from build123d import *

# Parameters (mm, degrees)
SKETCH1_W           = 508
SKETCH1_H           = 546.1
BOSS_EXTRUDE1_DEPTH = 1.6002
SKETCH2_R           = 6.35
CUT_EXTRUDE1_DEPTH  = 2.54
SKETCH3_R           = 3.2639
CUT_EXTRUDE3_DEPTH  = 373.927423422
SKETCH4_R           = 6.35
CUT_EXTRUDE4_DEPTH  = 2.54


with BuildPart() as part:
    # Sketch1 → Boss-Extrude1 (new body)
    with BuildSketch(Plane(origin=(0, 0, 0), x_dir=(1, 0, 0), z_dir=(0, 1, 0))):
        Rectangle(SKETCH1_W, SKETCH1_H)
    extrude(amount=BOSS_EXTRUDE1_DEPTH)

    # Sketch2 → Cut-Extrude1 (cut)
    with BuildSketch(Plane(origin=(0, 1.6002, 0), x_dir=(1, 0, 0), z_dir=(0, 1, 0))):
        with Locations(Location((215.9, 222.25, 0), (0, 0, 270))):
            Circle(SKETCH2_R)
        with Locations(Location((215.9, -171.45, 0), (0, 0, 270))):
            Circle(SKETCH2_R)
        with Locations(Location((-215.9, 222.25, 0), (0, 0, 270))):
            Circle(SKETCH2_R)
        with Locations(Location((-215.9, -171.45, 0), (0, 0, 270))):
            Circle(SKETCH2_R)
    extrude(amount=-CUT_EXTRUDE1_DEPTH, mode=Mode.SUBTRACT)

    # Sketch3 → Cut-Extrude3 (cut, through all)
    with BuildSketch(Plane(origin=(0, 1.6002, 0), x_dir=(1, 0, 0), z_dir=(0, 1, 0))):
        with Locations(Location((-241.3, 222.25, 0), (0, 0, 270))):
            Circle(SKETCH3_R)
        with Locations(Location((-241.3, 133.35, 0), (0, 0, 270))):
            Circle(SKETCH3_R)
        with Locations(Location((-241.3, 44.45, 0), (0, 0, 270))):
            Circle(SKETCH3_R)
        with Locations(Location((-241.3, -44.45, 0), (0, 0, 270))):
            Circle(SKETCH3_R)
        with Locations(Location((-241.3, -133.35, 0), (0, 0, 270))):
            Circle(SKETCH3_R)
        with Locations(Location((-241.3, -222.25, 0), (0, 0, 270))):
            Circle(SKETCH3_R)
        with Locations(Location((241.3, 222.25, 0), (0, 0, 90))):
            Circle(SKETCH3_R)
        with Locations(Location((241.3, 133.35, 0), (0, 0, 90))):
            Circle(SKETCH3_R)
        with Locations(Location((241.3, 44.45, 0), (0, 0, 90))):
            Circle(SKETCH3_R)
        with Locations(Location((241.3, -44.45, 0), (0, 0, 90))):
            Circle(SKETCH3_R)
        with Locations(Location((241.3, -133.35, 0), (0, 0, 90))):
            Circle(SKETCH3_R)
        with Locations(Location((241.3, -222.25, 0), (0, 0, 90))):
            Circle(SKETCH3_R)
    extrude(amount=-CUT_EXTRUDE3_DEPTH, mode=Mode.SUBTRACT)

    # Sketch4 → Cut-Extrude4 (cut)
    with BuildSketch(Plane(origin=(0, 1.6002, 0), x_dir=(1, 0, 0), z_dir=(0, 1, 0))):
        with Locations(Location((107.95, 25.4, 0), (0, 0, 270))):
            Circle(SKETCH4_R)
        with Locations(Location((-107.95, 25.4, 0), (0, 0, 270))):
            Circle(SKETCH4_R)
    extrude(amount=-CUT_EXTRUDE4_DEPTH, mode=Mode.SUBTRACT)


solid = part.part
CAD build for the part. Positions are in the model's coordinates, mm. Coordinates: 2 decimals unless noted, no trailing zeros. Loops run counter-clockwise (first coordinate to the right, second up) from the corner with the lowest first, then second, coordinate; pieces in that order, holes last. Notation, with made-up numbers: (84, 13) - (135, 13) arc R32 cw to (135, 49) - close; hole circle Ø8 at (3.25, 77.5). An arc over 180 degrees is marked (long way). Write item = value, one per line. Start each with the question number.
Q1. Cut at A-A, the plane x = -107.95. List the corners of the cut face in (y, z).
Q2. Drill centre lines: L1, parallel to X at y = 0.4, z = -222.25; L2, parallel to X at y = 1.05, z = 222.25; L3, parallel to X at y = 0.45, z = -221.5. Where is each one in solid material? Low to high.
Q3. Pull direction X, two halves, no side cores. Call faces 1 (the flat face through (-4, 1.6, -4)), 2 (the cylindrical face through (101.75, 0.81, -26.78)): pulls with the +X half, pulls with the -X half, needs draft (parallel to the pull), parting line crosses it, or undercut.
Q4. Flat gauge pins, fed straight in: pin 1 Ø10.5 at (x, z) = (241.3, 222.25) entering from -Y; pin 2 Ø11.5 at (x, z) = (-215.9, 171.45) entering from -Y. Where does each tip first touch, or does it go through?
Computed:
q1.outline = (0, -273.05) - (1.6, -273.05) - (1.6, -31.75) - (0, -31.75) - close; (0, -19.05) - (1.6, -19.05) - (1.6, 273.05) - (0, 273.05) - close
q2.L1 = -254 to -244.56, -238.04 to -222.25, -209.55 to 209.55, 222.25 to 238.04, 244.56 to 254
q2.L2 = -254 to -244.56, -238.04 to 238.04, 244.56 to 254
q2.L3 = -254 to -244.48, -238.12 to -222.21, -209.59 to 209.59, 222.21 to 238.12, 244.48 to 254
q3.face_1 = needs draft
q3.face_2 = undercut
q4.pin_1 = 0
q4.pin_2 = through
